Part model, mm, in its own coordinate system. Face numbers are marked on the shaded views. A direction names the side the tool comes from. Round coordinates to 2 decimals unless told otherwise and drop trailing zeros. Write each loop counter-clockwise with the first axis right and the second up, starting at its lowest first coordinate (ties: lowest second). Pieces come first, ordered by that corner, then holes. Notation, with made-up numbers: M -35,-36.75 L 12,-36.75 A18 ccw 12,-22.75 Z; hole C 43,0 d10. An arc over 180 degrees is marked long. Use one line per item in the form item = value. Start each with the question number.
Item 1: Cut at D-D, the plane x = 145. Give the cut face in (y, z), then the cut area to 3 significant figures.
Item 2: Cut at B-B, the plane x = 80. Give the cut face in (y, z), then the cut area to 3 significant figures.
Item 3: Cut at A-A, the plane z = 18.5. Give the cut face in (x, y), then the cut area to 3 significant figures.
Item 4: Which spindle directions (+Z, -Z, +X, -X, +Y, -Y) get a long thin tool onto all of the face, cutting with end or side? Do the marked faces 1, 2 and 3. Say none if no direction does.
Item 5: Flat gauge pins, fed straight in: pin 1 Ø1 at (x, y) = (59, 72) entering from +Z; pin 2 Ø12 at (x, y) = (135.5, 126) entering from +Z; pin 3 Ø2 at (x, y) = (57, 79.5) entering from -Z; pin 4 Ø3 at (x, z) = (21.5, 37.5) entering from +Y. Where does each tip first touch, or does it go through?
Item 6: Cut at C-C, the plane y = 129. Give the cut face in (x, z), then the cut area to 3 significant figures.
Item 7: Probe L1, parallel to Y at x = 80, z = 17; L2, parallel to Y at x = 80, z = 7; L3, parallel to Z at x = 16.5, y = 19. List the from-to ranges inside material, lowest first.
Item 8: Mould opens along X. For the marked faces 4, 5, 6 and 7 say: +X half, -X half, draft (parallel to the pull), parting line (faces both ways), or undercut.
from build123d import *

# Parameters (mm, degrees)
EXTRUDE_1_DEPTH          = 40
CUT_EXTRUDE_1_DEPTH      = 217.333076528
CUT_EXTRUDE_1_DEPTH_BACK = 217.333076528
SKETCH_4_W               = 70
SKETCH_4_H               = 20
EXTRUDE_2_DEPTH          = 15
SKETCH_5_3_R             = 50
SKETCH_5_3_R_2           = 29
EXTRUDE_3_DEPTH          = 25


with BuildPart() as part:
    # Sketch 1 → Extrude 1 (new body)
    with BuildSketch(Plane(origin=(0, 0, 0), x_dir=(1, 0, 0), z_dir=(0, 1, 0))):
        with BuildLine():
            Line((160, 0), (0, 0))
            Line((0, 0), (0, -140))
            Line((0, -140), (30, -140))
            ThreePointArc((30, -140), (80, -90), (130, -140))
            Line((130, -140), (160, -140))
            Line((160, -140), (160, 0))
        make_face()
    extrude(amount=EXTRUDE_1_DEPTH)

    # Sketch 4 → Cut-Extrude 1 (cut, two sides: drawn at the far end of the back side and taken through both)
    with BuildSketch(Plane.ZY.offset(-CUT_EXTRUDE_1_DEPTH_BACK)):
        with Locations((70, 10)):
            Rectangle(SKETCH_4_W, SKETCH_4_H)
    extrude(amount=CUT_EXTRUDE_1_DEPTH + CUT_EXTRUDE_1_DEPTH_BACK, mode=Mode.SUBTRACT)

    # Sketch 5 → Extrude 2 (add)
    with BuildSketch(Plane(origin=(0, 0, 0), x_dir=(-1, 0, 0), z_dir=(0, 0, -1))):
        with BuildLine():
            Line((-80, 70), (-80, 40))
            Line((-80, 40), (0, 40))
            Line((0, 40), (-32.659713859, 136.090286141))
            ThreePointArc((-32.659713859, 136.090286141), (-30.669409556, 128.154314593), (-30, 120))
            ThreePointArc((-30, 120), (-44.644660941, 84.644660941), (-80, 70))
        make_face()
        with BuildLine():
            Line((-160, 40), (-80, 40))
            Line((-80, 40), (-80, 70))
            ThreePointArc((-80, 70), (-120.647966167, 90.883976122), (-127.340286141, 136.090286141))
            Line((-127.340286141, 136.090286141), (-160, 40))
        make_face()
    extrude(amount=-EXTRUDE_2_DEPTH)

    # Sketch 5_3 → Extrude 3 (add)
    with BuildSketch(Plane(origin=(0, 0, 0), x_dir=(-1, 0, 0), z_dir=(0, 0, -1))):
        with Locations((-80, 120)):
            Circle(SKETCH_5_3_R)
        with Locations((-80, 120)):
            Circle(SKETCH_5_3_R_2, mode=Mode.SUBTRACT)
    extrude(amount=-EXTRUDE_3_DEPTH)


solid = part.part
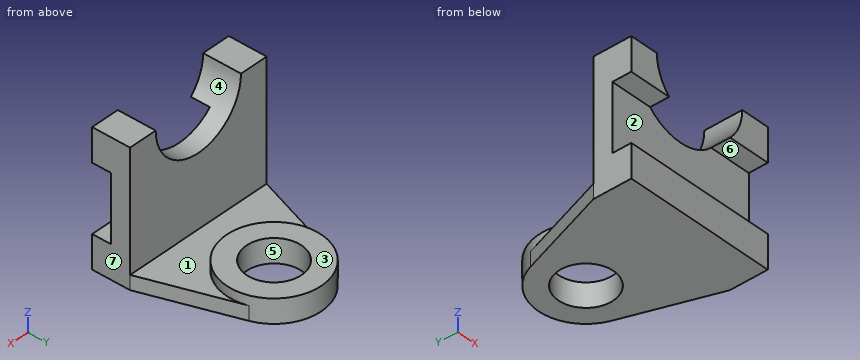
Model answer:
q1.outline = M 0,0 L 84.13,0 L 84.13,15 L 40,15 L 40,140 L 0,140 L 0,105 L 20,105 L 20,35 L 0,35 Z
q1.area = 4,860 mm²
q2.outline = M 0,0 L 91,0 L 91,25 L 70,25 L 70,15 L 40,15 L 40,90 L 20,90 L 20,35 L 0,35 Z; M 149,0 L 170,0 L 170,25 L 149,25 Z
q2.area = 4,000 mm²
q3.outline = M 0,0 L 160,0 L 160,40 L 0,40 Z; C 80,120 d100; hole C 80,120 d58
q3.area = 11,600 mm²
q4.face_1 = +Z
q4.face_2 = +X, -X, -Y
q4.face_3 = +Z, +X, -X, +Y
q5.pin_1 = 15
q5.pin_2 = 25
q5.pin_3 = 0
q5.pin_4 = 40
q6.outline = M 30.25,0 L 52.43,0 L 52.43,25 L 30.82,25 L 30.82,15 L 30.25,15 Z; M 107.57,0 L 129.75,0 L 129.75,15 L 129.18,15 L 129.18,25 L 107.57,25 Z
q6.area = 1,100 mm²
q7.L1 = 0 to 40, 70 to 91, 149 to 170
q7.L2 = 0 to 91, 149 to 170
q7.L3 = 0 to 35, 105 to 140
q8.face_4 = undercut
q8.face_5 = undercut
q8.face_6 = draft
q8.face_7 = +X half
